Could you check a few things on this model? Use its own coordinates, in mm. Coordinates: 2 decimals unless noted, no trailing zeros. Loops run counter-clockwise (first coordinate to the right, second up) from the corner with the lowest first, then second, coordinate; pieces in that order, holes last. Notation, with made-up numbers: M -4,-29 L 3,-29 A21 ccw 3,5 Z; hole C 38,-35 d10. An arc over 180 degrees is marked long. Use one line per item in the form item = value. Start each with the question number.
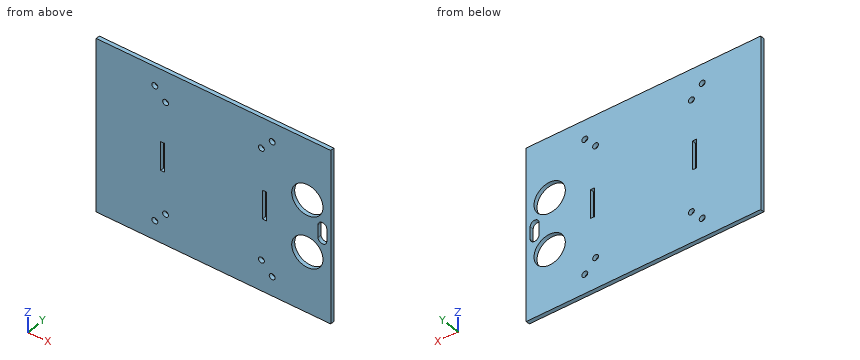
```python
from build123d import *

# Parameters (mm, degrees)
SKETCH_1_W          = 120
SKETCH_1_H          = 90
SKETCH_1_R          = 1.5
SKETCH_1_W_2        = 2
SKETCH_1_H_2        = 15
EXTRUDE_1_DEPTH     = 2
SKETCH_2_R          = 8
CUT_EXTRUDE_1_DEPTH = 3


with BuildPart() as part:
    # 草圖1 → 填料-伸長1 (new body)
    with BuildSketch(Plane(origin=(0, 0, 0), x_dir=(1, 0, 0), z_dir=(0, 1, 0))):
        Rectangle(SKETCH_1_W, SKETCH_1_H)
        with Locations((-30, 35)):
            Circle(SKETCH_1_R, mode=Mode.SUBTRACT)
        with Locations((30, 35)):
            Circle(SKETCH_1_R, mode=Mode.SUBTRACT)
        with Locations((30, -35)):
            Circle(SKETCH_1_R, mode=Mode.SUBTRACT)
        with Locations((-30, -35)):
            Circle(SKETCH_1_R, mode=Mode.SUBTRACT)
        with Locations((24.5, 29)):
            Circle(SKETCH_1_R, mode=Mode.SUBTRACT)
        with Locations((24.5, -29)):
            Circle(SKETCH_1_R, mode=Mode.SUBTRACT)
        with Locations((-24.5, 29)):
            Circle(SKETCH_1_R, mode=Mode.SUBTRACT)
        with Locations((-24.5, -29)):
            Circle(SKETCH_1_R, mode=Mode.SUBTRACT)
        with Locations((-26, 0)):
            Rectangle(SKETCH_1_W_2, SKETCH_1_H_2, mode=Mode.SUBTRACT)
        with Locations((26, 0)):
            Rectangle(SKETCH_1_W_2, SKETCH_1_H_2, mode=Mode.SUBTRACT)
    extrude(amount=EXTRUDE_1_DEPTH)

    # 草圖2 → 除料-伸長1 (cut, through all)
    with BuildSketch(Plane(origin=(0, 2, 0), x_dir=(1, 0, 0), z_dir=(0, 1, 0))):
        with Locations((48, 13.48)):
            Circle(SKETCH_2_R)
        with Locations((48, -13.48)):
            Circle(SKETCH_2_R)
        with BuildLine():
            Line((53.45, -3.25), (53.45, 3.25))
            ThreePointArc((53.45, 3.25), (55.7, 5.5), (57.95, 3.25))
            Line((57.95, 3.25), (57.95, -3.25))
            ThreePointArc((57.95, -3.25), (55.7, -5.5), (53.45, -3.25))
        make_face()
    extrude(amount=-CUT_EXTRUDE_1_DEPTH, mode=Mode.SUBTRACT)


solid = part.part
```
Item 1: Please list where these lines run through material, in increasing order: line 1 along Z through (x, y) = (-30, 0.75); line 2 along X through (y, z) = (1.2, -29); line 3 along X through (y, z) = (1.95, -2.5).
Item 2: I want a section at D-D (z = 20). Write out the boundary of the cut face in (x, y).
Item 3: I want a section at B-B (y = 1.6). Count the separate pieces of the cut face and the enclosed holes in it, plus the area to 3 significant figures.
Item 4: I want a section at A-A (z = 35). Write out the boundary of the cut face in (x, y), plus the area to 3 significant figures.
Item 5: I want a section at C-C (x = 48). Write out the boundary of the cut face in (y, z), plus the area to 3 significant figures.
Worked answers:
q1.line_1 = -45 to -36.5, -33.5 to 33.5, 36.5 to 45
q1.line_2 = -60 to -26, -23 to 23, 26 to 60
q1.line_3 = -60 to -27, -25 to 25, 27 to 53.45, 57.95 to 60
q2.outline = M -60,0 L 43.36,0 L 43.36,2 L -60,2 Z; M 52.64,0 L 60,0 L 60,2 L 52.64,2 Z
q3.separate_pieces = 1
q3.enclosed_holes = 13
q3.area = 10,200 mm²
q4.outline = M -60,0 L -31.5,0 L -31.5,2 L -60,2 Z; M -28.5,0 L 28.5,0 L 28.5,2 L -28.5,2 Z; M 31.5,0 L 60,0 L 60,2 L 31.5,2 Z
q4.area = 228 mm²
q5.outline = M 0,-45 L 2,-45 L 2,-21.48 L 0,-21.48 Z; M 0,-5.48 L 2,-5.48 L 2,5.48 L 0,5.48 Z; M 0,21.48 L 2,21.48 L 2,45 L 0,45 Z
q5.area = 116 mm²
